```python
from build123d import *

# Parameters (mm, degrees)
SKETCH1_R           = 1.5
BOSS_EXTRUDE1_DEPTH = 2.25
FILLET1_R           = 1
FILLET2_R           = 0.25


with BuildPart() as part:
    # Sketch1 → Boss-Extrude1 (new body)
    with BuildSketch(Plane(origin=(0, 0, 0), x_dir=(1, 0, 0), z_dir=(0, 1, 0))):
        Polygon((2.7, -1.558845727), (2.7, 1.558845727), (0, 3.117691454), (-2.7, 1.558845727), (-2.7, -1.558845727), (0, -3.117691454), align=None)
        Circle(SKETCH1_R, mode=Mode.SUBTRACT)
    extrude(amount=BOSS_EXTRUDE1_DEPTH)

    # Fillet1
    fillet1_edges = [part.edges().sort_by_distance(p)[0] for p in [
        (0, 1.125, 3.117691454),
        (-2.7, 1.125, 1.558845727),
        (-2.7, 1.125, -1.558845727),
        (0, 1.125, -3.117691454),
        (2.7, 1.125, -1.558845727),
        (2.7, 1.125, 1.558845727),
    ]]
    fillet(fillet1_edges, radius=FILLET1_R)

    # Fillet2
    fillet2_edges = [part.edges().sort_by_distance(p)[0] for p in [
        (-1.5, 0, 0),
        (-1.5, 2.25, 0),
        (-1.35, 0, -2.33826859),
        (-1.35, 2.25, -2.33826859),
        (1.35, 0, 2.33826859),
        (-1.35, 0, 2.33826859),
        (-2.7, 0, 0),
        (1.35, 0, -2.33826859),
        (2.7, 0, 0),
        (0, 0, 2.962990915),
        (2.566025404, 0, 1.481495458),
        (2.566025404, 0, -1.481495458),
        (-2.566025404, 0, 1.481495458),
        (-2.566025404, 0, -1.481495458),
        (0, 0, -2.962990915),
        (1.35, 2.25, -2.33826859),
        (1.35, 2.25, 2.33826859),
        (2.7, 2.25, 0),
        (-2.7, 2.25, 0),
        (-1.35, 2.25, 2.33826859),
        (0, 2.25, 2.962990915),
        (2.566025404, 2.25, 1.481495458),
        (2.566025404, 2.25, -1.481495458),
        (-2.566025404, 2.25, 1.481495458),
        (-2.566025404, 2.25, -1.481495458),
        (0, 2.25, -2.962990915),
    ]]
    fillet(fillet2_edges, radius=FILLET2_R)


solid = part.part
```
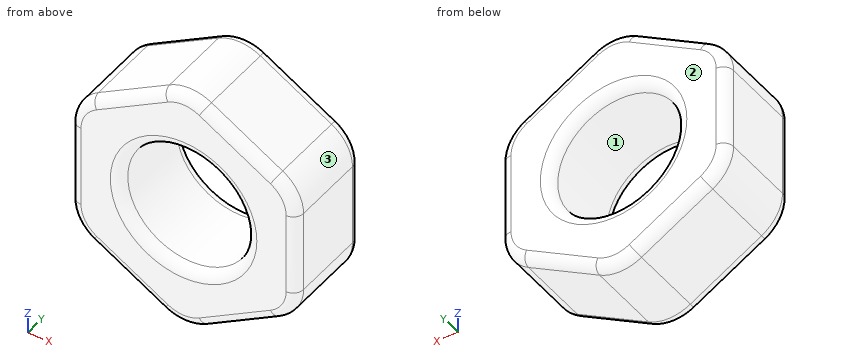
Could you check a few things on this model? Use its own coordinates, in mm. Face numbers are marked on the shaded views. Round coordinates to 2 decimals unless told otherwise and drop trailing zeros. Write each loop counter-clockwise with the first axis right and the second up, starting at its lowest first coordinate (ties: lowest second). Pieces come first, ordered by that corner, then holes. Notation, with made-up numbers: M 19,54.5 L 31,54.5 A17 cw 31,61.5 Z; hole C 53.25,69 d9. An arc over 180 degrees is marked long. Answer in a Markdown table with one row per item. Add a question column.
Q1. Imagine slicing it at B-B (x = 0). Please give me the cut outline in (y, z), then the cut area to 3 significant figures.
Q2. If we mould it in two halves opening along Z, with no side actions, what happens to the marked faces 1, 2 and 3? For each: +Z half, -Z half, draft (parallel to the pull), parting line (faces both ways), or undercut.
Q3. Imagine slicing it at C-C (y = 0.9). Please give me the cut outline in (x, z), then the cut area to 3 significant figures.
Q4. If I drill on line 1 (X direction, y = 1.25, z = 0); line 2 (Z direction, x = 0, y = 1.35); line 3 (Z direction, x = 1.25, y = 1.8), over which ranges is the centre line in solid material (lowest first)? Write a range as from..to.
Q5. Imagine slicing it at A-A (z = 0). Please give me the cut outline in (x, y), then the cut area to 3 significant figures.
Values:
| question | item | result |
|---|---|---|
| 1 | outline | M 0,-2.71 A0.25 ccw 0.25,-2.96 L 2,-2.96 A0.25 ccw 2.25,-2.71 L 2.25,-1.75 A0.25 ccw 2,-1.5 L 0.25,-1.5 A0.25 ccw 0,-1.75 Z; M 0,1.75 A0.25 ccw 0.25,1.5 L 2,1.5 A0.25 ccw 2.25,1.75 L 2.25,2.71 A0.25 ccw 2,2.96 L 0.25,2.96 A0.25 ccw 0,2.71 Z |
| 1 | area | 6.48 mm^2 |
| 2 | face 1 | undercut |
| 2 | face 2 | draft |
| 2 | face 3 | +Z half |
| 3 | outline | M -2.7,-0.98 A1 ccw -2.2,-1.85 L -0.5,-2.83 A1 ccw 0.5,-2.83 L 2.2,-1.85 A1 ccw 2.7,-0.98 L 2.7,0.98 A1 ccw 2.2,1.85 L 0.5,2.83 A1 ccw -0.5,2.83 L -2.2,1.85 A1 ccw -2.7,0.98 Z; hole C 0,0 d3 |
| 3 | area | 17.9 mm^2 |
| 4 | line 1 | -2.7..-1.5, 1.5..2.7 |
| 4 | line 2 | -2.96..-1.5, 1.5..2.96 |
| 4 | line 3 | -2.4..-0.83, 0.83..2.4 |
| 5 | outline | M -2.7,0.25 A0.25 ccw -2.45,0 L -1.75,0 A0.25 ccw -1.5,0.25 L -1.5,2 A0.25 ccw -1.75,2.25 L -2.45,2.25 A0.25 ccw -2.7,2 Z; M 1.5,0.25 A0.25 ccw 1.75,0 L 2.45,0 A0.25 ccw 2.7,0.25 L 2.7,2 A0.25 ccw 2.45,2.25 L 1.75,2.25 A0.25 ccw 1.5,2 Z |
| 5 | area | 5.29 mm^2 |
